```python
from build123d import *

# Parameters (mm, degrees)
EXTRUDE_1_DEPTH = 3
SKETCH_2_R      = 3.6
EXTRUDE_2_DEPTH = 2


with BuildPart() as part:
    # 草圖1 → 填料-伸長1 (new body)
    with BuildSketch(Plane(origin=(0, 0, 0), x_dir=(1, 0, 0), z_dir=(0, 1, 0))):
        with BuildLine():
            Line((-6.54186917, -3.868326222), (-6.54186917, -40.044486982))
            ThreePointArc((-6.54186917, -40.044486982), (0, -46.586356152), (6.54186917, -40.044486982))
            Line((6.54186917, -40.044486982), (6.54186917, -3.868326222))
            ThreePointArc((6.54186917, -3.868326222), (0, 7.6), (-6.54186917, -3.868326222))
        make_face()
        with BuildLine():
            Line((-2.6, -2.48997992), (-2.05, -14.677576073))
            ThreePointArc((-2.05, -14.677576073), (0, -16.637150357), (2.05, -14.677576073))
            Line((2.05, -14.677576073), (2.6, -2.48997992))
            ThreePointArc((2.6, -2.48997992), (0, 3.6), (-2.6, -2.48997992))
        make_face(mode=Mode.SUBTRACT)
    extrude(amount=EXTRUDE_1_DEPTH)

    # 草圖2 → 填料-伸長2 (add)
    with BuildSketch(Plane(origin=(0, 3, 0), x_dir=(1, 0, 0), z_dir=(0, 1, 0))):
        with BuildLine():
            Line((-6.451996083, -3.823839241), (-6.451996083, -40))
            ThreePointArc((-6.451996083, -40), (0, -46.451996083), (6.451996083, -40))
            Line((6.451996083, -40), (6.451996083, -3.823839241))
            ThreePointArc((6.451996083, -3.823839241), (0, 7.5), (-6.451996083, -3.823839241))
        make_face()
        Circle(SKETCH_2_R, mode=Mode.SUBTRACT)
    extrude(amount=EXTRUDE_2_DEPTH)


solid = part.part
```
The model under review builds one solid part; all positions refer to its coordinate system, in mm. A direction names the side the tool comes from. Give positions to 0.01 mm unless a question says otherwise; leave off trailing zeros. Loops run counter-clockwise (first coordinate to the right, second up) from the corner with the lowest first, then second, coordinate; pieces in that order, holes last. Notation, with made-up numbers: (12.25, -23.5) - (24.25, -23.5) arc R14 cw to (24.25, -11.5) - close; hole circle Ø10 at (69, -22.75). An arc over 180 degrees is marked (long way). Answer as a JSON object with one key per item and string values.
Q1. To check wall thickness, follow line 1 along X through (y, z) = (4.3, 0); line 2 along Z through (x, y) = (0, 3.95); line 3 along X through (y, z) = (1.5, 0). State the ranges of each line that lie inside material, in increasing order.
Worked out:
{"line 1": "x = -7.5 to -3.6, 3.6 to 7.5", "line 2": "z = -7.5 to -3.6, 3.6 to 46.45", "line 3": "x = -7.6 to -3.6, 3.6 to 7.6"}
Q2. Mouldability with a two-part tool opening along Z and no side actions: class faces 1 (the cylindrical face through (-0.044, 1.479, 16.637)), 2 (the cylindrical face through (0.221, 3.986, -7.497)), 3 (the cylindrical face through (-0.144, 1.479, 46.585)), 4 (the flat face through (2.32, 1.48, 8.67)) as +Z half, -Z half, draft (parallel to the pull), parting line (faces both ways), or undercut.
Worked out:
{"face 1": "undercut", "face 2": "parting line", "face 3": "+Z half", "face 4": "undercut"}
Q3. Add section C-C on z = 28.5. State the section outline as (x, y) points, plus the area to 3 significant figures.
Worked out:
{"outline": "(-6.54, 0) - (6.54, 0) - (6.54, 3) - (6.45, 3) - (6.45, 5) - (-6.45, 5) - (-6.45, 3) - (-6.54, 3) - close", "area": "65.1 mm^2"}
Q4. Insertion check: pin 1 (3 mm diameter, centred on y = 2, z = 34.5, fed in from -X); pin 2 (5.5 mm diameter, centred on x = 0.5, z = 7.5, fed in from -Y); pin 3 (1.5 mm diameter, centred on y = 2, z = 16, fed in from +X); pin 4 (1.5 mm diameter, centred on x = 5, y = 0.5, fed in from -Z). Each pin has a flat end and moves straight along its axis. Give the tip position at first contact, or say it passes through.
Worked out:
{"pin 1": "stops at x = -6.54", "pin 2": "stops at y = 0", "pin 3": "stops at x = 6.54", "pin 4": "stops at z = -6.3"}
Q5. Add section D-D on x = 4.25. State the section outline as (y, z) points, plus the area to 3 significant figures.
Worked out:
{"outline": "(0, -6.3) - (3, -6.3) - (3, -6.18) - (5, -6.18) - (5, 44.85) - (3, 44.85) - (3, 45.02) - (0, 45.02) - close", "area": "256 mm^2"}
Q6. For faces 5 (the flat face through (0, 3, 9)), 6 (the flat face through (6.452, 4, 22)), 7 (the flat face through (-6.452, 4, 22)), 8 (the cylindrical face through (-0.14, 3.99, 46.45)), list the 3-axis set-ups (+Z, -Z, +X, -X, +Y, -Y) from which the entire face can be reached by the end or side of a thin tool; tool diameter is ignored.
Worked out:
{"face 5": "-Y", "face 6": "+Z, +X, +Y", "face 7": "+Z, -X, +Y", "face 8": "+Z, +Y"}
Q7. Add section B-B on x = 0. State the section outline as (y, z) points.
Worked out:
{"outline": "(0, -7.6) - (3, -7.6) - (3, -7.5) - (5, -7.5) - (5, -3.6) - (0, -3.6) - close; (0, 16.64) - (3, 16.64) - (3, 3.6) - (5, 3.6) - (5, 46.45) - (3, 46.45) - (3, 46.59) - (0, 46.59) - close"}
Q8. Add section A-A on z = 0. State the section outline as (x, y) points, plus the area to 3 significant figures.
Worked out:
{"outline": "(-7.6, 0) - (-3.6, 0) - (-3.6, 5) - (-7.5, 5) - (-7.5, 3) - (-7.6, 3) - close; (3.6, 0) - (7.6, 0) - (7.6, 3) - (7.5, 3) - (7.5, 5) - (3.6, 5) - close", "area": "39.6 mm^2"}
